```python
from build123d import *

# Parameters (mm, degrees)
SKETCH001_W     = 7.8
SKETCH001_H     = 7.8
PAD_DEPTH       = 4.5
POCKET_DEPTH    = 5
POCKET001_DEPTH = 5
POCKET002_DEPTH = 5


with BuildPart() as part:
    # Sketch → Revolution (revolve)
    with BuildSketch(Plane.XZ):
        with BuildLine():
            Line((0, 0), (0, 2))
            Line((0, 2), (-2.1, 2))
            ThreePointArc((-2.1, 2), (-2.382843, 1.882843), (-2.5, 1.6))
            Line((-2.5, 1.6), (-2.5, 0))
            Line((-2.5, 0), (0, 0))
        make_face()
    revolve(axis=Axis((0, 0, 0), (0, 0, 1)))

    # Sketch001 → Pad (new body)
    with BuildSketch(Plane.XY):
        Rectangle(SKETCH001_W, SKETCH001_H)
    extrude(amount=-PAD_DEPTH)

    # Sketch002 → Pocket (cut, symmetric)
    with BuildSketch(Plane.YZ):
        with BuildLine():
            ThreePointArc((-1.4, -1.45), (-2.2, -2.25), (-1.4, -3.05))
            Line((-1.4, -3.05), (1.4, -3.05))
            ThreePointArc((1.4, -3.05), (2.2, -2.25), (1.4, -1.45))
            Line((-1.4, -1.45), (1.4, -1.45))
        make_face()
    extrude(amount=POCKET_DEPTH, both=True, mode=Mode.SUBTRACT)

    # Sketch003 → Pocket001 (cut)
    with BuildSketch(Plane.XZ):
        Polygon((1.1, -5.9), (-1.1, -5.9), (-1.1, -2.9), (-5.1, -2.9), (-5.1, -1.7), (1.1, -1.7), align=None)
    extrude(amount=POCKET001_DEPTH, mode=Mode.SUBTRACT)

    # Sketch004 → Pocket002 (cut)
    with BuildSketch(Plane.XZ):
        Polygon((-1.1, -1.7), (-1.1, -6.7), (1.1, -6.7), (1.1, -2.9), (5.1, -2.9), (5.1, -1.7), align=None)
    extrude(amount=-POCKET002_DEPTH, mode=Mode.SUBTRACT)


solid = part.part
```
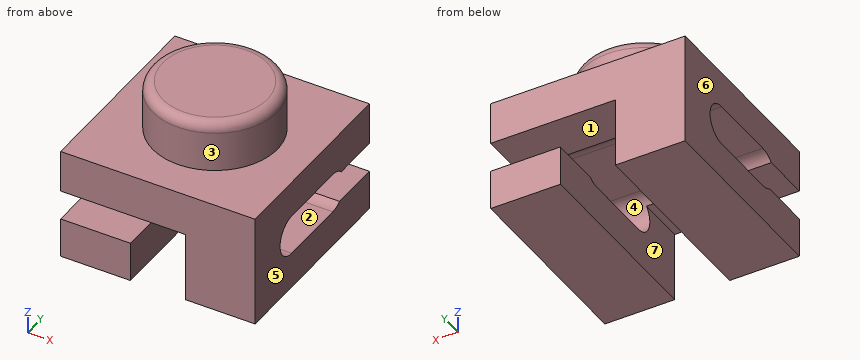
Work out the finished part from the listing and answer in its coordinate system (mm). Face numbers are marked on the shaded views. A direction names the side the tool comes from. Give positions to 0.01 mm unless a question says otherwise; leave off trailing zeros. Write each loop counter-clockwise with the first axis right and the second up, starting at its lowest first coordinate (ties: lowest second). Pieces come first, ordered by that corner, then holes. Notation, with made-up numbers: (-10, 57) -> (33, 57) arc R24 ccw to (33, 95) -> close; hole circle Ø3 at (10.25, 55). An arc over 180 degrees is marked (long way). Write each question's results on one line, items separated by ' | '.
1. Find section B-B on z = -2.25. Determine the outline of the cut face in (x, y).
Data:
outline: (-3.9, 2.2) -> (-1.1, 2.2) -> (-1.1, 3.9) -> (-3.9, 3.9) -> close; (1.1, -3.9) -> (3.9, -3.9) -> (3.9, -2.2) -> (1.1, -2.2) -> close
2. Straight lines are drawn through the part: L1, parallel to Z at x = -3, y = 0.5; L2, parallel to Z at x = 2.75, y = 3.75; L3, parallel to X at y = 1.5, z = -3.5. For each, find the intervals that lie inside material, in ascending order.
Data:
L1: -4.5 to -3.05, -1.45 to 0 | L2: -4.5 to -2.9, -1.7 to 0 | L3: -3.9 to -1.1, 1.1 to 3.9
3. Find section D-D on y = 1.25. Give the number of separate pieces and of enclosed holes in the cut face, and give its area (3 significant figures).
Data:
separate pieces: 3 | enclosed holes: 0 | area: 28.0 mm^2
4. Find section C-C on x = 2.75. Determine the outline of the cut face in (y, z), and give its area (3 significant figures).
Data:
outline: (-3.9, -4.5) -> (3.9, -4.5) -> (3.9, -2.9) -> (1.87, -2.9) arc R0.8 cw to (1.4, -3.05) -> (-1.4, -3.05) arc R0.8 cw to (-1.4, -1.45) -> (1.4, -1.45) arc R0.8 cw to (1.98, -1.7) -> (3.9, -1.7) -> (3.9, 0) -> (-3.9, 0) -> close | area: 26.5 mm^2
5. A tool of negligible diameter and unlimited length cuts with its end or side. For the marked faces 1, 2 and 3, from which of +Z, -Z, +X, -X, +Y, -Y can it reach the whole face along a straight path? Write none if from no direction.
Data:
face 1: +X, +Y | face 2: +X, -X | face 3: +Z
6. This flat-tipped pin is pushed along its axis until it touches: pin 1 Ø1 at (x, y) = (-2.5, -3) entering from +Z. Where does it stop, or does it pass through?
Data:
pin 1: z = 0
7. Determine the mould class of the marked faces 4, 5, 6 and 7 for opening direction X: +X half, -X half, draft (parallel to the pull), parting line (faces both ways), or undercut.
Data:
face 4: draft | face 5: +X half | face 6: -X half | face 7: undercut
8. Find section A-A on y = 3.75. Determine the outline of the cut face in (x, z), and give its area (3 significant figures).
Data:
outline: (-3.9, -4.5) -> (-1.1, -4.5) -> (-1.1, -1.7) -> (3.9, -1.7) -> (3.9, 0) -> (-3.9, 0) -> close; (1.1, -4.5) -> (3.9, -4.5) -> (3.9, -2.9) -> (1.1, -2.9) -> close | area: 25.6 mm^2
